```python
from build123d import *

# Parameters (mm, degrees)
SKETCH1_R                = 7.75
SKETCH1_R_2              = 3
BOSS_EXTRUDE3_DEPTH      = 3
BOSS_EXTRUDE4_DEPTH      = 3
BOSS_EXTRUDE4_DEPTH_BACK = 3
SKETCH3_R                = 3
SKETCH3_R_2              = 1.7025
CUT_EXTRUDE2_DEPTH       = 0.5


with BuildPart() as part:
    # Sketch1 → Boss-Extrude3 (new body)
    with BuildSketch(Plane.XY):
        with BuildLine():
            Line((8.434915556, -5.371424351), (21.165047264, 14.249110995))
            ThreePointArc((21.165047264, 14.249110995), (21.364152327, 19.357269814), (16.970562748, 21.970562748))
            Line((16.970562748, 21.970562748), (-17.47367286, 22.673506332))
            ThreePointArc((-17.47367286, 22.673506332), (-22.032126076, 20.135047844), (-21.848877926, 14.920674696))
            Line((-21.848877926, 14.920674696), (-8.342416793, -5.513989668))
            ThreePointArc((-8.342416793, -5.513989668), (0.084971894, -9.999638982), (8.434915556, -5.371424351))
        make_face()
        Circle(SKETCH1_R, mode=Mode.SUBTRACT)
        with Locations((-17.67766953, 17.67766953)):
            Circle(SKETCH1_R_2, mode=Mode.SUBTRACT)
        with Locations((16.970562748, 16.970562748)):
            Circle(SKETCH1_R_2, mode=Mode.SUBTRACT)
    extrude(amount=BOSS_EXTRUDE3_DEPTH)

    # Sketch3 → Boss-Extrude4 (add, two sides: drawn at the far end of the back side and taken through both)
    # profile 1 of 2: a face of its own
    with BuildSketch(Plane.XY.offset(3).offset(-BOSS_EXTRUDE4_DEPTH_BACK)):
        with Locations((-17.67766953, 17.67766953)):
            Circle(SKETCH3_R)
        with Locations((-17.67766953, 17.67766953)):
            Circle(SKETCH3_R_2, mode=Mode.SUBTRACT)
    # profile 2 of 2: a face of its own
    with BuildSketch(Plane.XY.offset(3).offset(-BOSS_EXTRUDE4_DEPTH_BACK)):
        with Locations((16.970562748, 16.970562748)):
            Circle(SKETCH3_R)
        with Locations((16.970562748, 16.970562748)):
            Circle(SKETCH3_R_2, mode=Mode.SUBTRACT)
    extrude(amount=BOSS_EXTRUDE4_DEPTH + BOSS_EXTRUDE4_DEPTH_BACK)

    # Sketch4 → Cut-Extrude2 (cut)
    with BuildSketch(Plane(origin=(0, 0, 0), x_dir=(-1, 0, 0), z_dir=(0, 0, -1))):
        with BuildLine():
            Line((-0.665908197, 13.903438218), (0.066062957, 13.903438218))
            add(Edge.make_bspline(
                [(0.066062957, 13.903438218), (0.114446028, 13.903266485), (0.207500301, 13.902936196), (0.341679481, 13.897725107), (0.46494151, 13.890473447), (0.577468889, 13.879407223), (0.679213477, 13.864734748), (0.770277246, 13.847438327), (0.850657534, 13.827725347), (0.921032238, 13.803161419), (0.984541929, 13.775453681), (1.04374179, 13.743616981), (1.099937859, 13.708005833), (1.152754525, 13.667683209), (1.202650778, 13.623374504), (1.24972075, 13.575035117), (1.293299299, 13.522255149), (1.333116584, 13.465368105), (1.369406835, 13.405524238), (1.401479805, 13.342641383), (1.427561597, 13.27667581), (1.450607657, 13.208580863), (1.467206987, 13.137383112), (1.478751578, 13.063775679), (1.487204076, 12.987499458), (1.487690054, 12.93568078), (1.487937957, 12.909247512)],
                knots=[0, 0, 0, 0, 1.749336639, 3.364467119, 4.854658419, 6.213483162, 7.451590619, 8.570285859, 9.5643256, 10.440900261, 11.26203566, 12.067320669, 12.869050712, 13.665104639, 14.467235401, 15.27997916, 16.102287765, 16.939272006, 17.78853747, 18.631303466, 19.488103222, 20.351255419, 21.228522269, 22.127379805, 23.044756219, 24, 24, 24, 24], degree=3))
            add(Edge.make_bspline(
                [(1.487937957, 12.909247512), (1.487293995, 12.881657254), (1.486031303, 12.827557785), (1.479229754, 12.748090078), (1.46679866, 12.672060935), (1.447969959, 12.599692959), (1.426328814, 12.530085447), (1.397551641, 12.4645227), (1.365073758, 12.402051204), (1.326500725, 12.343554641), (1.284168705, 12.287733687), (1.234937457, 12.236727048), (1.181996409, 12.187793312), (1.122369551, 12.143997521), (1.058685292, 12.102378362), (0.989678292, 12.064660321), (0.915798913, 12.029895252), (0.863858052, 12.010507848), (0.837296932, 12.000593666)],
                knots=[0, 0, 0, 0, 1.099860209, 2.156625411, 3.176576793, 4.16617041, 5.135385252, 6.078461593, 7.016046972, 7.938469504, 8.868247731, 9.803980173, 10.76021508, 11.73834243, 12.748633912, 13.790971185, 14.870363756, 16, 16, 16, 16], degree=3))
            Line((0.837296932, 12.000593666), (1.644989239, 10.403438218))
            Line((1.644989239, 10.403438218), (0.946671932, 10.403438218))
            Line((0.946671932, 10.403438218), (0.175437957, 11.929079243))
            Line((0.175437957, 11.929079243), (-0.037703068, 11.929079243))
            Line((-0.037703068, 11.929079243), (-0.037703068, 10.403438218))
            Line((-0.037703068, 10.403438218), (-0.665908197, 10.403438218))
            Line((-0.665908197, 10.403438218), (-0.665908197, 13.903438218))
        make_face()
        with BuildLine():
            Line((-0.037703068, 12.557284371), (0.206988438, 12.557284371))
            add(Edge.make_bspline(
                [(0.206988438, 12.557284371), (0.236904009, 12.557621301), (0.294185898, 12.558266448), (0.376564779, 12.561258908), (0.45138445, 12.568469257), (0.51896621, 12.577579265), (0.579650126, 12.588098083), (0.632894918, 12.60317219), (0.679521008, 12.619324476), (0.718975873, 12.639397578), (0.752685204, 12.662225049), (0.781791054, 12.688157623), (0.805865765, 12.718171276), (0.82568048, 12.751450365), (0.841094174, 12.788289236), (0.85234499, 12.828283482), (0.858632532, 12.871888689), (0.859355935, 12.90198222), (0.859732829, 12.917660974)],
                knots=[0, 0, 0, 0, 1.688639943, 3.233382647, 4.650958383, 5.928841754, 7.082724185, 8.122798841, 9.049171256, 9.863274652, 10.613301712, 11.341792392, 12.054588806, 12.776240173, 13.521029143, 14.301969904, 15.115324896, 16, 16, 16, 16], degree=3))
            add(Edge.make_bspline(
                [(0.859732829, 12.917660974), (0.859020277, 12.936210085), (0.857620601, 12.972646377), (0.843731463, 13.02510186), (0.821622957, 13.073652999), (0.791318249, 13.118080428), (0.75315341, 13.157028578), (0.709356247, 13.191361683), (0.658981509, 13.218509733), (0.612338294, 13.236416298), (0.56990387, 13.247129981), (0.531608141, 13.255113722), (0.487261456, 13.260772029), (0.436830336, 13.266773671), (0.380443332, 13.270665431), (0.317793101, 13.273505641), (0.249059573, 13.27466771), (0.201145777, 13.275039203), (0.176139079, 13.275233089)],
                knots=[0, 0, 0, 0, 1.020303359, 2.004196876, 2.966617323, 3.9489082, 4.950758222, 5.960522915, 7.003732012, 8.091992268, 8.70421221, 9.413913587, 10.24622431, 11.166358409, 12.212345909, 13.359657661, 14.621978493, 16, 16, 16, 16], degree=3))
            Line((0.176139079, 13.275233089), (-0.037703068, 13.275233089))
            Line((-0.037703068, 13.275233089), (-0.037703068, 12.557284371))
        make_face(mode=Mode.SUBTRACT)
    extrude(amount=-CUT_EXTRUDE2_DEPTH, mode=Mode.SUBTRACT)


solid = part.part
```
Could you check a few things on this model? Use its own coordinates, in mm. A direction names the side the tool comes from. Coordinates: 2 decimals unless noted, no trailing zeros. Write each loop counter-clockwise with the first axis right and the second up, starting at its lowest first coordinate (ties: lowest second). Pieces come first, ordered by that corner, then holes. Notation, with made-up numbers: (-34, 45.25) -> (-30, 45.25) arc R17 ccw to (-30, 78.25) -> close; hole circle Ø7 at (-20.5, -6.5). An arc over 180 degrees is marked (long way). Write item = value, one per line. Start each with the question number.
(1) Will these pins go through, and if not, where does the flat tip stop? pin 1 (2 mm diameter, centred on x = -17.68, y = 17.68, fed in from +Z); pin 2 (0.6 mm diameter, centred on y = 12, z = 0.5, fed in from -X); pin 3 (0.6 mm diameter, centred on y = 13, z = 0, fed in from +X); pin 4 (16.5 mm diameter, centred on x = 0, y = 13.5, fed in from +Z).
(2) I want a section at A-A (x = -5). Please give me the cut outline in (y, z).
(3) I want a section at D-D (z = 4). Please give me the cut outline in (x, y) (1 decimal).
(4) We'd pull the mould along Y, two halves only. Please class faces 1 (the face through (15.62, 15.935, 2.958)), 2 (the face through (21.4, 19.29, 1.48)), 3 (the face through (14.71, 4.3, 1.48)): released by +Y, released by -Y, zero draft, split by the parting line, or undercut.
(5) I need wall thicknesses on line 1 (X direction, y = 17, z = 1.25); line 2 (Z direction, x = -3.5, y = 9); line 3 (Y direction, x = 4.5, z = 1). Which ranges of each line are inside material? Lowest first, please. Write a range as [from, to].
(6) Which directions (+Z, -Z, +X, -X, +Y, -Y) give clear straight access to the entire face, cutting with the end or side of a thin tool? Please do faces 4 (the face through (19, 17, 6)), 5 (the face through (-0.2, 12.2, 0.5)), 6 (the face through (-20.058, 15.852, 4.479)).
(7) I want a section at B-B (y = -1.5). Please give me the cut outline in (x, z), plus the area to 3 significant figures.
(8) I want a section at C-C (z = 1.25). Give the number of separate pieces and of enclosed holes in the cut face, plus the area to 3 significant figures.
Result set:
q1.pin_1 = through
q1.pin_2 = -20.12
q1.pin_3 = 20.55
q1.pin_4 = 3
q2.outline = (-8.66, 0) -> (-5.92, 0) -> (-5.92, 3) -> (-8.66, 3) -> close; (5.92, 0) -> (22.42, 0) -> (22.42, 3) -> (5.92, 3) -> close
q3.outline = circle Ø6 at (-17.7, 17.7); circle Ø6 at (17, 17); hole circle Ø3.4 at (-17.7, 17.7); hole circle Ø3.4 at (17, 17)
q4.face_1 = undercut
q4.face_2 = split by the parting line
q4.face_3 = released by -Y
q5.line_1 = [-22.63, -19.24], [-16.12, 15.27], [18.67, 21.97]
q5.line_2 = [0, 3]
q5.line_3 = [-8.93, -6.31], [6.31, 22.23]
q6.face_4 = +Z, +X, -X, +Y, -Y
q6.face_5 = -Z
q6.face_6 = +Z
q7.outline = (-11, 0) -> (-7.6, 0) -> (-7.6, 3) -> (-11, 3) -> close; (7.6, 0) -> (10.95, 0) -> (10.95, 3) -> (7.6, 3) -> close
q7.area = 20.2 mm2
q8.separate_pieces = 1
q8.enclosed_holes = 3
q8.area = 779 mm2
